from build123d import *

# Parameters (mm, degrees)
SKETCH002_W     = 42.5
SKETCH002_H     = 28
PAD_DEPTH       = 3
SKETCH_R        = 2
POCKET_DEPTH    = 5
SKETCH001_R     = 2
POCKET001_DEPTH = 5
SKETCH003_W     = 42.5
SKETCH003_H     = 2.5
PAD001_DEPTH    = 20


with BuildPart() as part:
    # Sketch002 → Pad (new body)
    with BuildSketch(Plane.XY):
        with Locations((13.25, -6)):
            Rectangle(SKETCH002_W, SKETCH002_H)
    extrude(amount=PAD_DEPTH)

    # Sketch → Pocket (cut)
    with BuildSketch(Plane.XY):
        Circle(SKETCH_R)
    extrude(amount=POCKET_DEPTH, mode=Mode.SUBTRACT)

    # Sketch001 → Pocket001 (cut)
    with BuildSketch(Plane.XY):
        with Locations((26.5, 0)):
            Circle(SKETCH001_R)
    extrude(amount=POCKET001_DEPTH, mode=Mode.SUBTRACT)

    # Sketch003 → Pad001 (join)
    with BuildSketch(Plane.XY):
        with Locations((13.25, -18.75)):
            Rectangle(SKETCH003_W, SKETCH003_H)
    extrude(amount=-PAD001_DEPTH)


solid = part.part
Read the model definition and answer for the solid it produces. Units are mm, in the model's axes. A direction names the side the tool comes from. Round coordinates to 2 decimals unless told otherwise and drop trailing zeros. Write each loop counter-clockwise with the first axis right and the second up, starting at its lowest first coordinate (ties: lowest second). Pieces come first, ordered by that corner, then holes.
Q1. Find section D-D on z = -3. Determine the outline of the cut face in (x, y).
Values:
outline: (-8, -20) - (34.5, -20) - (34.5, -17.5) - (-8, -17.5) - close
Q2. Find section C-C on x = 7. Determine the outline of the cut face in (y, z), and give its area (3 significant figures).
Values:
outline: (-20, -20) - (-17.5, -20) - (-17.5, 0) - (8, 0) - (8, 3) - (-20, 3) - close
area: 134 mm2
Q3. Flat-ended cylindrical pins translate along their axes: P1, Ø6, axis at x = 10.5, z = -8, coming from the +Y side; P2, Ø7.5, axis at x = 22.5, y = 0, coming from the -Z side. Find the tip coordinate at first contact, or state that the pin passes through.
Values:
P1: stops at y = -17.5
P2: stops at z = 0
Q4. Find section A-A on y = 0. Determine the outline of the cut face in (x, z).
Values:
outline: (-8, 0) - (-2, 0) - (-2, 3) - (-8, 3) - close; (2, 0) - (24.5, 0) - (24.5, 3) - (2, 3) - close; (28.5, 0) - (34.5, 0) - (34.5, 3) - (28.5, 3) - close
Q5. The mould has two halves that part along Y. Classify faces 3 (the face through (13, 8, 1)), 4 (the face through (0, -2, 1)), 5 (the face through (13, -5, 0)): released by +Y, released by -Y, zero draft, split by the parting line, or undercut.
Values:
face 3: released by +Y
face 4: undercut
face 5: zero draft
Q6. A tool of negligible diameter and unlimited length cuts with its end or side. For faces 1 (the face through (-8, -9, 1)), 2 (the face through (13, -17.5, -10)), from which of +Z, -Z, +X, -X, +Y, -Y can it reach the whole face along a straight path? Write none if from no direction.
Values:
face 1: +Z, -Z, -X, +Y, -Y
face 2: -Z, +X, -X, +Y
Q7. Find section B-B on x = 0. Determine the outline of the cut face in (y, z), and give its area (3 significant figures).
Values:
outline: (-20, -20) - (-17.5, -20) - (-17.5, 0) - (-2, 0) - (-2, 3) - (-20, 3) - close; (2, 0) - (8, 0) - (8, 3) - (2, 3) - close
area: 122 mm2
Q8. Straight lines are drawn through the part: line 1 (X direction, y = 0, z = 2.1); line 2 (Y direction, x = 0, z = 1.05); line 3 (Y direction, x = 3, z = -15.75). For each, find the intervals that lie inside material, in ascending order.
Values:
line 1: x = -8 to -2, 2 to 24.5, 28.5 to 34.5
line 2: y = -20 to -2, 2 to 8
line 3: y = -20 to -17.5
